from build123d import *

# Parameters (mm, degrees)
EXTRUDE_START   = -30
SKETCH_1_R      = 8.666666667
EXTRUDE_1_DEPTH = 30


with BuildPart() as part:
    # 草图1 → 凸台-拉伸1 (new body)
    with BuildSketch(Plane.XY.offset(EXTRUDE_START)):
        with BuildLine():
            Line((47.521768078, 23), (37.478231922, 23))
            ThreePointArc((37.478231922, 23), (30.40716411, 20.071067812), (27.478231922, 13))
            Line((27.478231922, 13), (27.478231922, 0))
            Line((27.478231922, 0), (57.521768078, 0))
            Line((57.521768078, 0), (57.521768078, 13))
            ThreePointArc((57.521768078, 13), (54.59283589, 20.071067812), (47.521768078, 23))
        make_face()
        with Locations((42.5, 11.5)):
            Circle(SKETCH_1_R, mode=Mode.SUBTRACT)
    extrude(amount=-EXTRUDE_1_DEPTH)


solid = part.part
CAD build for the part. Positions are in the model's coordinates, mm. Coordinates: 2 decimals unless noted, no trailing zeros. Order: outer loops, then holes, each group sorted by start corner. A loop starts at its lowest first (then second) coordinate and runs counter-clockwise, first axis right, second up.
Item 1: Two-plate mould, pull along Y, no slides. Class faces 1 (the face through (40.62, 3.04, -44.79)), 2 (the face through (42, 1, -60)), 3 (the face through (42, 0, -45)): +Y half, -Y half, draft (parallel to the pull), parting line (faces both ways), or undercut.
Check sheet entries:
face 1: undercut
face 2: draft
face 3: -Y half
Item 2: Drill centre lines: L1, parallel to Y at x = 42.5, z = -40; L2, parallel to X at y = 13.25, z = -47; L3, parallel to Y at x = 47, z = -37. Where is each one in solid material? Low to high.
Check sheet entries:
L1: y = 0 to 2.83, 20.17 to 23
L2: x = 27.48 to 34.01, 50.99 to 57.52
L3: y = 0 to 4.09, 18.91 to 23
Item 3: Band-saw the part on B-B on x = 42.5. List the corners of the cut face in (y, z), plus the area to 3 significant figures.
Check sheet entries:
outline: (0, -60) - (2.83, -60) - (2.83, -30) - (0, -30) - close; (20.17, -60) - (23, -60) - (23, -30) - (20.17, -30) - close
area: 170 mm2
Item 4: Band-saw the part on A-A on z = -46.25. List the corners of the cut face in (x, y).
Check sheet entries:
outline: (27.48, 0) - (57.52, 0) - (57.52, 13) arc R10 ccw to (47.52, 23) - (37.48, 23) arc R10 ccw to (27.48, 13) - close; hole circle Ø17.33 at (42.5, 11.5)
Item 5: Band-saw the part on C-C on y = 11.5. List the corners of the cut face in (x, z), plus the area to 3 significant figures.
Check sheet entries:
outline: (27.48, -60) - (33.83, -60) - (33.83, -30) - (27.48, -30) - close; (51.17, -60) - (57.52, -60) - (57.52, -30) - (51.17, -30) - close
area: 381 mm2
Item 6: Band-saw the part on D-D on y = 21.5. List the corners of the cut face in (x, z), plus the area to 3 significant figures.
Check sheet entries:
outline: (32.21, -60) - (52.79, -60) - (52.79, -30) - (32.21, -30) - close
area: 617 mm2
Item 7: Pin check, flat tips, straight feed: pin 1 Ø4 at (y, z) = (18, -49) entering from -X; pin 2 Ø6 at (x, z) = (54, -42) entering from +Y. Stop position of each tip, or through.
Check sheet entries:
pin 1: stops at x = 27.94
pin 2: stops at y = 22.38
